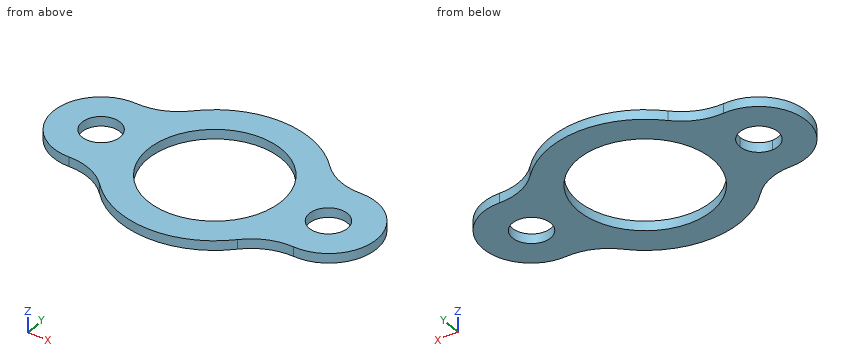
```python
from build123d import *

# Parameters (mm, degrees)
F0_R     = 44.45
F0_R_2   = 12.7
F1_DEPTH = 6.35


with BuildPart() as f1:
    # F0 (on Top) → F1 (new body)
    with BuildSketch(Plane.XY):
        with BuildLine():
            ThreePointArc((-76.2, -12.7), (-67.219744, -8.980256), (-63.5, 0))
            ThreePointArc((-63.5, 0), (-85.180256, 8.980256), (-76.2, -12.7))
        make_face()
        with BuildLine():
            ThreePointArc((-46.136719, 43.630874), (-59.347524, 34.564632), (-75.117614, 31.731545))
            ThreePointArc((-75.117614, 31.731545), (-107.95, 0), (-75.117614, -31.731545))
            ThreePointArc((-75.117614, -31.731545), (-59.347524, -34.564632), (-46.136719, -43.630874))
            ThreePointArc((-46.136719, -43.630874), (0.097237, -63.499926), (46.270126, -43.489372))
            ThreePointArc((46.270126, -43.489372), (59.493096, -34.366174), (75.300953, -31.504125))
            ThreePointArc((75.300953, -31.504125), (108.108105, 0.323178), (75.111252, 31.953768))
            ThreePointArc((75.111252, 31.953768), (59.286566, 34.721254), (46.009287, 43.765232))
            ThreePointArc((46.009287, 43.765232), (-0.092589, 63.499932), (-46.136719, 43.630874))
        make_face()
        with BuildLine():
            ThreePointArc((-76.2, -12.7), (-85.180256, 8.980256), (-63.5, 0))
            ThreePointArc((-63.5, 0), (-67.219744, -8.980256), (-76.2, -12.7))
        make_face(mode=Mode.SUBTRACT)
        Circle(F0_R, mode=Mode.SUBTRACT)
        with Locations((76.2, 0)):
            Circle(F0_R_2, mode=Mode.SUBTRACT)
    extrude(amount=-F1_DEPTH)


solid = f1.part
```
Verification items for the finished model (mm, model axes). Give positions to 0.01 mm unless a question says otherwise; leave off trailing zeros. Order: outer loops, then holes, each group sorted by start corner. A loop starts at its lowest first (then second) coordinate and runs counter-clockwise, first axis right, second up. Notation, with made-up numbers: M 55,56 L 65,56 A23 ccw 65,77 Z; hole C 75.5,61 d7. An arc over 180 degrees is marked long. Return JSON: item names as keys, results as strings. Group by question number.
1) Section check A-A on x = 0. Record the cut outline in (y, z).
2) Section check D-D on y = 51. Record the cut outline in (x, z).
3) Go/stop test with flat-tipped pins: pin 1 Ø3 at (y, z) = (-14.5, -3.5) entering from +X; pin 2 Ø2 at (x, z) = (6.5, -2.5) entering from -Y; pin 3 Ø6 at (x, y) = (-53.5, 41) entering from -Z; pin 4 Ø15 at (x, y) = (76.2, 0) entering from -Z. Record where each tip stops, or that it passes through.
4) Scan lines: line 1 (Y direction, x = -76.2, z = -4); line 2 (Y direction, x = 0, z = -3); line 3 (X direction, y = 5.5, z = -5.5). Record each from-to range of solid material in increasing order.
5) Section check C-C on y = -47. Record the cut outline in (x, z).
6) Section check B-B on y = 15. Record the cut outline in (x, z), and give its area (4 significant figures).
Answer block:
{
 "1": {"outline": "M -63.5,-6.35 L -44.45,-6.35 L -44.45,0 L -63.5,0 Z; M 44.45,-6.35 L 63.5,-6.35 L 63.5,0 L 44.45,0 Z"},
 "2": {"outline": "M -37.83,-6.35 L 37.83,-6.35 L 37.83,0 L -37.83,0 Z"},
 "3": {"pin 1": "stops at x = 105.22", "pin 2": "stops at y = -63.26", "pin 3": "stops at z = -6.35", "pin 4": "passes through"},
 "4": {"line 1": "y = -31.75 to -12.7, 12.7 to 31.75", "line 2": "y = -63.5 to -44.45, 44.45 to 63.5", "line 3": "x = -107.47 to -87.65, -64.75 to -44.11, 44.11 to 64.75, 87.65 to 107.67"},
 "5": {"outline": "M -42.7,-6.35 L 42.7,-6.35 L 42.7,0 L -42.7,0 Z"},
 "6": {"outline": "M -104.18,-6.35 L -41.84,-6.35 L -41.84,0 L -104.18,0 Z; M 41.84,-6.35 L 104.46,-6.35 L 104.46,0 L 41.84,0 Z", "area": "793.5 mm^2"}
}
